from build123d import *

# Parameters (mm, degrees)
SKETCH1_R           = 14.975
SKETCH1_R_2         = 1.7
BOSS_EXTRUDE2_DEPTH = 5
CUT_EXTRUDE1_REACH  = 164.524
SKETCH3_R           = 1.7


with BuildPart() as part:
    # Sketch1 → Boss-Extrude2 (new body)
    with BuildSketch(Plane(origin=(0, 0, 0), x_dir=(1, 0, 0), z_dir=(0, 1, 0))):
        with BuildLine():
            Line((12.756485957, 16.650005737), (-5.812603326, 30.876807241))
            ThreePointArc((-5.812603326, 30.876807241), (-10.178871966, 35.493803021), (-12.876419651, 41.247426954))
            Line((-12.876419651, 41.247426954), (-21.13456265, 70.088423369))
            ThreePointArc((-21.13456265, 70.088423369), (-24.125041887, 85.243134658), (-22.456551163, 100.599709115))
            ThreePointArc((-22.456551163, 100.599709115), (-19.558480324, 114.843106453), (-18.020623668, 129.29676271))
            ThreePointArc((-18.020623668, 129.29676271), (-18.441772746, 133.226047543), (-20.116399197, 136.805470974))
            ThreePointArc((-20.116399197, 136.805470974), (-25.866377757, 144.615905974), (-32.098124488, 152.047627243))
            ThreePointArc((-32.098124488, 152.047627243), (-38.706331156, 153.910886754), (-43.194615771, 148.715173848))
            Line((-43.194615771, 148.715173848), (-50.932711484, 96.056215067))
            ThreePointArc((-50.932711484, 96.056215067), (-51.118515181, 89.191813761), (-50.383474997, 82.364351257))
            Line((-50.383474997, 82.364351257), (-44.824720745, 40.290812443))
            ThreePointArc((-44.824720745, 40.290812443), (-42.928869469, 32.33094735), (-39.452930017, 24.92341407))
            Line((-39.452930017, 24.92341407), (-17.977463078, -10.80562105))
            ThreePointArc((-17.977463078, -10.80562105), (13.973815194, -15.642350012), (12.756485957, 16.650005737))
        make_face()
        with Locations(Location((0, 0, 0), (0, 0, 270))):
            Circle(SKETCH1_R, mode=Mode.SUBTRACT)
        with Locations(Location((-28.930848813, 17.123276905, 0), (0, 0, 270))):
            Circle(SKETCH1_R_2, mode=Mode.SUBTRACT)
    extrude(amount=BOSS_EXTRUDE2_DEPTH)

    # Sketch3 → Cut-Extrude1 (cut, up to next)
    with BuildSketch(Plane(origin=(0, 5, 0), x_dir=(1, 0, 0), z_dir=(0, 1, 0)), mode=Mode.PRIVATE) as cut_extrude1_sk1:
        with Locations(Location((-35, 131, 0), (0, 0, 270))):
            Circle(SKETCH3_R)
    cut_extrude1_tool1 = extrude(cut_extrude1_sk1.sketch, amount=-CUT_EXTRUDE1_REACH, mode=Mode.PRIVATE) & part.part
    # Sketch3 → Cut-Extrude1 (cut, up to next)
    with BuildSketch(Plane(origin=(0, 5, 0), x_dir=(1, 0, 0), z_dir=(0, 1, 0)), mode=Mode.PRIVATE) as cut_extrude1_sk2:
        with Locations(Location((-35, 106, 0), (0, 0, 270))):
            Circle(SKETCH3_R)
    cut_extrude1_tool2 = extrude(cut_extrude1_sk2.sketch, amount=-CUT_EXTRUDE1_REACH, mode=Mode.PRIVATE) & part.part
    add(cut_extrude1_tool1.solids().sort_by_distance((-35, 5, -131))[0], mode=Mode.SUBTRACT)
    add(cut_extrude1_tool2.solids().sort_by_distance((-35, 5, -106))[0], mode=Mode.SUBTRACT)


solid = part.part
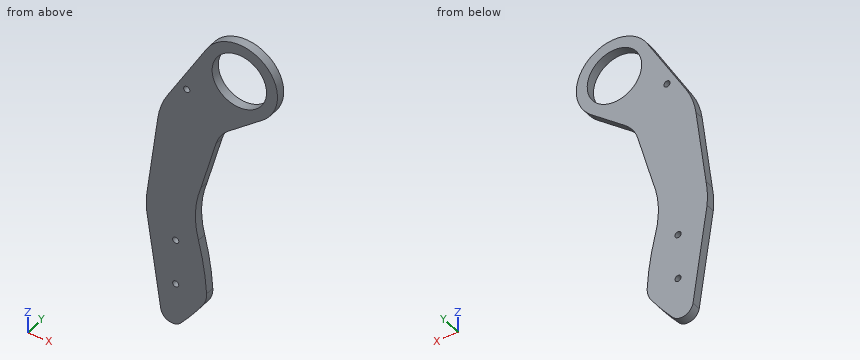
Source: CAD feature listing. Evaluate the final solid. Frame: model axes, mm. Round coordinates to 2 decimals unless told otherwise and drop trailing zeros. Loops run counter-clockwise (first coordinate to the right, second up) from the corner with the lowest first, then second, coordinate; pieces in that order, holes last.
Q1. Section A-A, the plane x = 5. Return loops of the section in (y, z), plus the area to 3 significant figures.
Q2. Section D-D, the plane z = -102.5. Return loops of the section in (x, y), plus the area to 3 significant figures.
Q3. Section B-B, the plane y = 2.95. Return loops of the section in (x, z) (3 decimals), plus the area to 3 significant figures.
Q4. Ray query, line 1 (Z direction, x = 9, y = 4.55); line 2 (X direction, y = 4.2, z = -11.5); line 3 (X direction, y = 2.65, z = -131). Return the intervals inside material, ascending.
Q5. Section C-C, the plane z = -131. Return loops of the section in (x, y).
Q6. First-contact query: P1, Ø3, axis at y = 3, z = -64.5, coming from the +X side; P2, Ø1, axis at x = -42, y = 2, coming from the -Z side; P3, Ø8, axis at x = -11.5, z = -61, coming from the -Y side. Flat tips, straight axial feed; report the tip coordinate or a pass-through.
Solutions:
1. outline: (0, -22.59) - (5, -22.59) - (5, -14.12) - (0, -14.12) - close; (0, 14.12) - (5, 14.12) - (5, 20.37) - (0, 20.37) - close
1. area: 73.7 mm2
2. outline: (-49.99, 0) - (-21.99, 0) - (-21.99, 5) - (-49.99, 5) - close
2. area: 140 mm2
3. outline: (-50.933, -96.056) - (-43.195, -148.715) arc R6.396 ccw to (-32.098, -152.048) arc R153.5 ccw to (-20.116, -136.805) arc R12 ccw to (-18.021, -129.297) arc R153.5 ccw to (-22.457, -100.6) arc R51.167 cw to (-21.135, -70.088) - (-12.876, -41.247) arc R20 cw to (-5.813, -30.877) - (12.756, -16.65) arc R20.975 ccw (long way) to (-17.977, 10.806) - (-39.453, -24.923) arc R40 ccw to (-44.825, -40.291) - (-50.383, -82.364) arc R51.167 ccw to start; hole circle Ø3.4 at (-35, -131); hole circle Ø3.4 at (-35, -106); hole circle Ø3.4 at (-28.931, -17.123); hole circle Ø29.95 at (0, 0)
3. area: 4,710 mm2
4. line 1: z = -19.53 to -11.97, 11.97 to 18.95
4. line 2: x = -31.38 to -9.59, 9.59 to 17.54
4. line 3: x = -45.8 to -36.7, -33.3 to -18.04
5. outline: (-45.8, 0) - (-36.7, 0) - (-36.7, 5) - (-45.8, 5) - close; (-33.3, 0) - (-18.04, 0) - (-18.04, 5) - (-33.3, 5) - close
6. P1: stops at x = -19.1
6. P2: stops at z = -152.19
6. P3: passes through
